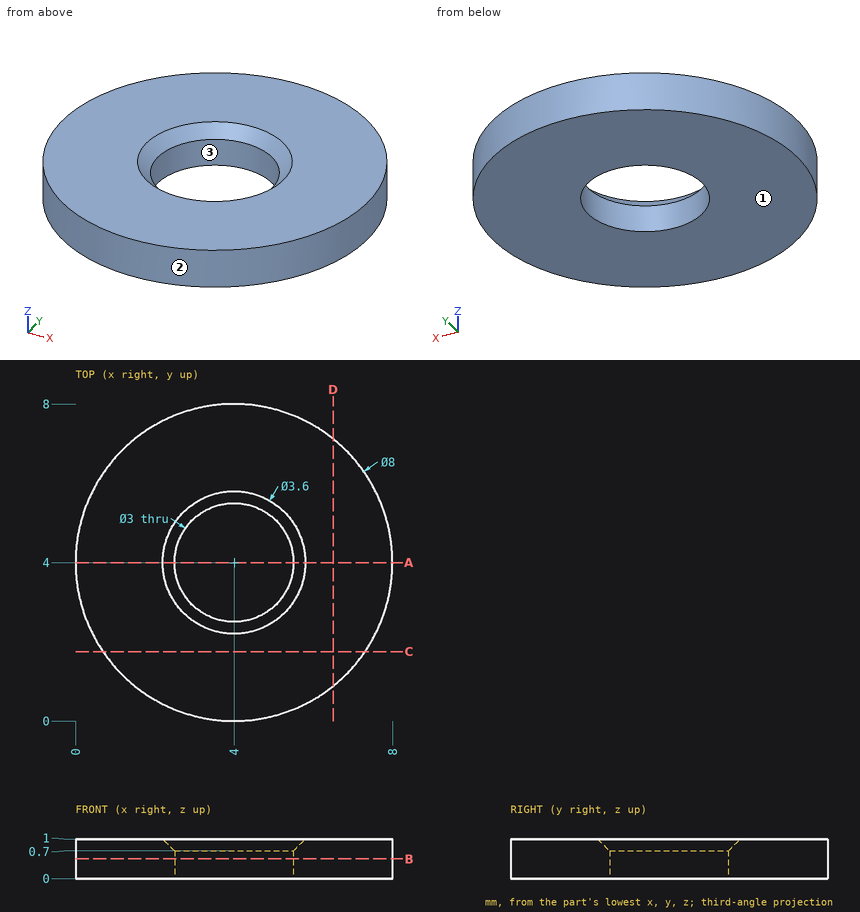
Study the drawing (mm; zero at the part's minimum x, y, z) and answer. Round coordinates to 2 decimals unless told otherwise and drop trailing zeros. Order: outer loops, then holes, each group sorted by start corner. A loop starts at its lowest first (then second) coordinate and runs counter-clockwise, first axis right, second up. Notation, with made-up numbers: (-10, 17.25) - (43, 17.25) arc R25 cw to (43, 34.25) - close; hole circle Ø6 at (54, 11.25). An arc over 180 degrees is marked (long way). Use one line per item in the form item = value. Start each with the question number.
(1) The part is cut by section C-C (y = 1.75). Give the vertices of the cut face in (x, z).
(2) The part is cut by section A-A (y = 4). Give the vertices of the cut face in (x, z), then the cut area to 3 significant figures.
(3) Determine the mould class of the marked faces 1, 2 and 3 for opening direction X: +X half, -X half, draft (parallel to the pull), parting line (faces both ways), or undercut.
(4) Find the intervals of material crossed by line 1 along Y through (x, z) = (4, 0.4); line 2 along X through (y, z) = (3, 0.35); line 3 along Y through (x, z) = (3.5, 0.5), in increasing order. Write a range as from..to.
(5) The part is cut by section B-B (z = 0.5). Give the vertices of the cut face in (x, y).
(6) The part is cut by section D-D (x = 6.5). Give the vertices of the cut face in (y, z).
Checked values:
q1.outline = (0.69, 0) - (7.31, 0) - (7.31, 1) - (0.69, 1) - close
q2.outline = (0, 0) - (2.5, 0) - (2.5, 0.7) - (2.2, 1) - (0, 1) - close; (5.5, 0) - (8, 0) - (8, 1) - (5.8, 1) - (5.5, 0.7) - close
q2.area = 4.91 mm^2
q3.face_1 = draft
q3.face_2 = parting line
q3.face_3 = undercut
q4.line_1 = 0..2.5, 5.5..8
q4.line_2 = 0.13..2.88, 5.12..7.87
q4.line_3 = 0.03..2.59, 5.41..7.97
q5.outline = circle Ø8 at (4, 4); hole circle Ø3 at (4, 4)
q6.outline = (0.88, 0) - (7.12, 0) - (7.12, 1) - (0.88, 1) - close
